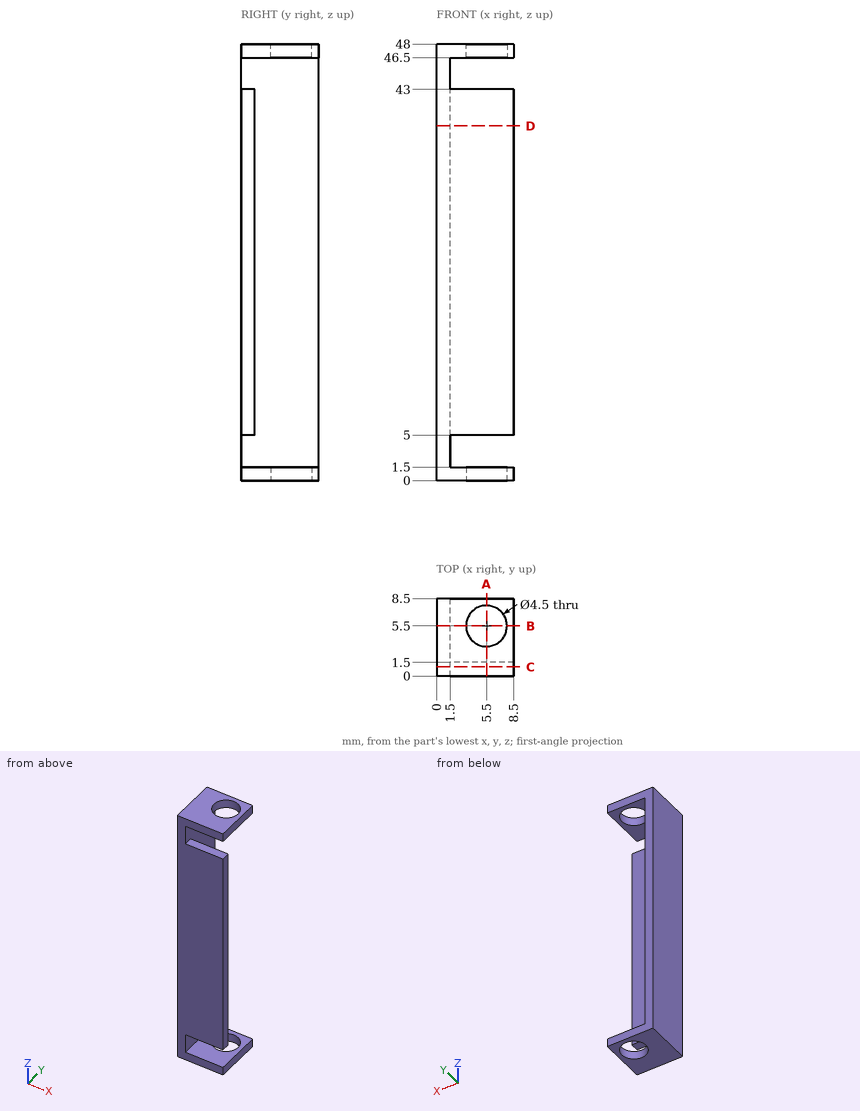
The drawing under review shows one solid part. Ordinate dimensions are in mm from its lowest x, y, z. Round coordinates to 2 decimals unless told otherwise and drop trailing zeros. Loops run counter-clockwise (first coordinate to the right, second up) from the corner with the lowest first, then second, coordinate; pieces in that order, holes last. Notation, with made-up numbers: (66, -9.75) -> (120, -9.75) arc R17 ccw to (120, 12.25) -> close; hole circle Ø10 at (-1, 69). An arc over 180 degrees is marked (long way). Answer in a Markdown table with one row per item.
1) Consider section A-A, the plane x = 5.5. Write out the cut boundary in (y, z).
Taken from the geometry:
| item | result |
|---|---|
| outline | (0, 0) -> (3.25, 0) -> (3.25, 1.5) -> (0, 1.5) -> close; (0, 5) -> (1.5, 5) -> (1.5, 43) -> (0, 43) -> close; (0, 46.5) -> (3.25, 46.5) -> (3.25, 48) -> (0, 48) -> close; (7.75, 0) -> (8.5, 0) -> (8.5, 1.5) -> (7.75, 1.5) -> close; (7.75, 46.5) -> (8.5, 46.5) -> (8.5, 48) -> (7.75, 48) -> close |
2) Wall thickness on line 1 along Z through (x, y) = (2, 1); line 2 along Z through (x, y) = (3, 8.25); line 3 along Y through (x, z) = (5.5, 47.65): over which ranges is each line inside the solid? List them lowest first.
Taken from the geometry:
| item | result |
|---|---|
| line 1 | z = 0 to 1.5, 5 to 43, 46.5 to 48 |
| line 2 | z = 0 to 1.5, 46.5 to 48 |
| line 3 | y = 0 to 3.25, 7.75 to 8.5 |
3) Consider section B-B, the plane y = 5.5. Write out the cut boundary in (x, z).
Taken from the geometry:
| item | result |
|---|---|
| outline | (0, 0) -> (3.25, 0) -> (3.25, 1.5) -> (1.5, 1.5) -> (1.5, 46.5) -> (3.25, 46.5) -> (3.25, 48) -> (0, 48) -> close; (7.75, 0) -> (8.5, 0) -> (8.5, 1.5) -> (7.75, 1.5) -> close; (7.75, 46.5) -> (8.5, 46.5) -> (8.5, 48) -> (7.75, 48) -> close |
4) For pin 1 Ø5 at (x, z) = (6.5, 8.5) entering from +Y; pin 2 Ø3.5 at (x, y) = (5.5, 5.5) entering from +Z, all flat-tipped, find the tip position at first contact; note any pin that passes through.
Taken from the geometry:
| item | result |
|---|---|
| pin 1 | stops at y = 1.5 |
| pin 2 | passes through |
5) Consider section D-D, the plane z = 39. Write out the cut boundary in (x, y), plus the area to 4 significant figures.
Taken from the geometry:
| item | result |
|---|---|
| outline | (0, 0) -> (8.5, 0) -> (8.5, 1.5) -> (1.5, 1.5) -> (1.5, 8.5) -> (0, 8.5) -> close |
| area | 23.25 mm² |
6) Consider section C-C, the plane y = 1. Write out the cut boundary in (x, z), plus the area to 3 significant figures.
Taken from the geometry:
| item | result |
|---|---|
| outline | (0, 0) -> (8.5, 0) -> (8.5, 1.5) -> (1.5, 1.5) -> (1.5, 5) -> (8.5, 5) -> (8.5, 43) -> (1.5, 43) -> (1.5, 46.5) -> (8.5, 46.5) -> (8.5, 48) -> (0, 48) -> close |
| area | 359 mm² |
